```python
from build123d import *

# Parameters (mm, degrees)
SKETCH2_R           = 7.62
SKETCH2_R_2         = 4.445
BOSS_EXTRUDE1_DEPTH = 2
CHAMFER1_SIZE       = 0.5


with BuildPart() as part:
    # Sketch1 → Revolve1 (revolve)
    with BuildSketch(Plane(origin=(0, 0, 0), x_dir=(0, 0, -1), z_dir=(1, 0, 0)), mode=Mode.PRIVATE) as revolve1_sk:
        Polygon((7.62, 2.5), (7.62, 5.5), (4.445, 5.5), (4.445, -5.5), (7.14375, -5.5), (7.14375, 1.5), (6.64375, 1.5), (6.64375, 2.5), align=None)
    revolve(revolve1_sk.sketch.rotate(Axis((0, 13.854588054, 0), (0, -1, 0)), 180), axis=Axis((0, 13.854588054, 0), (0, -1, 0)))  # turned: the seam where the file's is

    # Sketch2 → Boss-Extrude1 (add)
    with BuildSketch(Plane(origin=(0, 5.5, 0), x_dir=(1, 0, 0), z_dir=(0, 1, 0))):
        Polygon((4.487397232, 7.7724), (-4.487397232, 7.7724), (-8.974794464, 0), (-4.487397232, -7.7724), (4.487397232, -7.7724), (8.974794464, 0), align=None)
        with Locations(Location((0, 0, 0), (0, 0, 270))):  # turned: the seam where the file's is
            Circle(SKETCH2_R, mode=Mode.SUBTRACT)
        with Locations(Location((0, 0, 0), (0, 0, 270))):  # turned: the seam where the file's is
            Circle(SKETCH2_R)
        with Locations(Location((0, 0, 0), (0, 0, 270))):  # turned: the seam where the file's is
            Circle(SKETCH2_R_2, mode=Mode.SUBTRACT)
    extrude(amount=-BOSS_EXTRUDE1_DEPTH)

    # Chamfer1
    chamfer1_edges = [part.edges().sort_by_distance(p)[0] for p in [
        (0, -5.5, -7.14375),
    ]]
    chamfer(chamfer1_edges, length=CHAMFER1_SIZE)


solid = part.part
```
Part model, mm, in its own coordinate system. A direction names the side the tool comes from. Round coordinates to 2 decimals unless told otherwise and drop trailing zeros. Order: outer loops, then holes, each group sorted by start corner. A loop starts at its lowest first (then second) coordinate and runs counter-clockwise, first axis right, second up. Notation, with made-up numbers: M -32.5,-10 L 23.5,-10 A19 cw 23.5,-2 Z; hole C 32.5,-9.75 d8. An arc over 180 degrees is marked long. Answer in a Markdown table with one row per item. Add a question column.
Q1. Cut at A-A on x = 0. Give the cut face in (y, z) (3 decimals), and give its area (3 significant figures).
Q2. Pin check, flat tips, straight feed: pin 1 (3 mm diameter, centred on y = 4, z = -3.5, fed in from +X); pin 2 (1 mm diameter, centred on x = -7, z = 5.5, fed in from +Y); pin 3 (6 mm diameter, centred on y = 3, z = -3.5, fed in from -X). Stop position of each tip, or through.
Q3. 3-axis set-ups, long thin cutter, end or side, ignore diameter. For faces 1 (the face through (-1.996, 2.007, 6.337)), 2 (the face through (0, 5, -7.772)), 3 (the face through (-0.314, -1.704, -7.137)): which of +Z, -Z, +X, -X, +Y, -Y reach the whole face in a straight line?
Q4. Wall check: L1, parallel to X at y = 0, z = 0 (3 decimals); L2, parallel to X at y = 2, z = 0 (3 decimals); L3, parallel to Y at x = 7.25, z = -2.5. Give the ranges that are in metal, low to high. Write a range as from..to.
Q5. Mould opens along Y. For faces 4 (the face through (4.34, -5.5, 1.57)), 5 (the face through (6.7, 4.51, 3.94)), 6 (the face through (-7, 2.5, -1)) say: +Y half, -Y half, draft (parallel to the pull), parting line (faces both ways), or undercut.
Q6. Cut at B-B on y = -1. Give the cut face in (x, z) (1 decimal), and give its area (3 significant figures).
Established:
| question | item | result |
|---|---|---|
| 1 | outline | M -5.5,-6.644 L -5,-7.144 L 1.5,-7.144 L 1.5,-6.644 L 2.5,-6.644 L 2.5,-7.62 L 3.5,-7.62 L 3.5,-7.772 L 5.5,-7.772 L 5.5,-4.445 L -5.5,-4.445 Z; M -5.5,4.445 L 5.5,4.445 L 5.5,7.772 L 3.5,7.772 L 3.5,7.62 L 2.5,7.62 L 2.5,6.644 L 1.5,6.644 L 1.5,7.144 L -5,7.144 L -5.5,6.644 Z |
| 1 | area | 61.6 mm2 |
| 2 | pin 1 | stops at x = 7.82 |
| 2 | pin 2 | passes through |
| 2 | pin 3 | stops at x = -8.66 |
| 3 | face 1 | none |
| 3 | face 2 | -Z, +X, -X, +Y, -Y |
| 3 | face 3 | -Y |
| 4 | L1 | x = -7.144..-4.445, 4.445..7.144 |
| 4 | L2 | x = -6.644..-4.445, 4.445..6.644 |
| 4 | L3 | y = 3.5..5.5 |
| 5 | face 4 | -Y half |
| 5 | face 5 | draft |
| 5 | face 6 | undercut |
| 6 | outline | C 0,0 d14.3; hole C 0,0 d8.9 |
| 6 | area | 98.3 mm2 |
